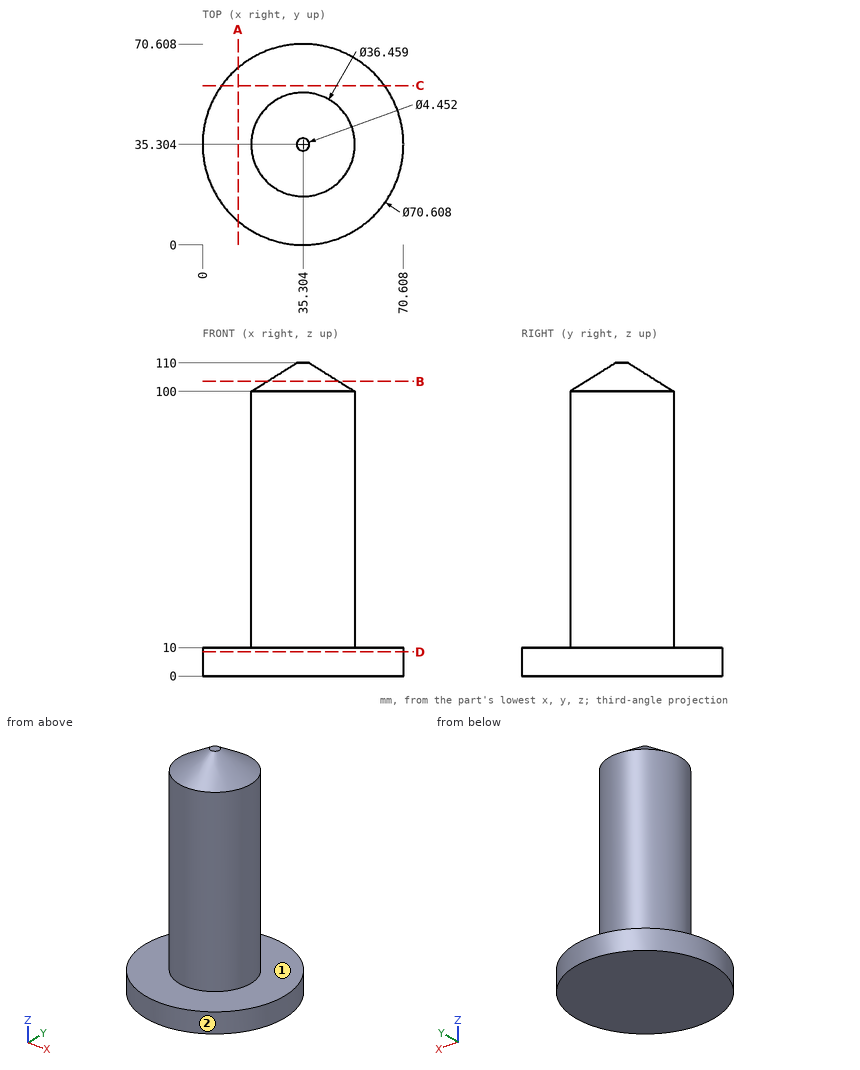
Can you work these out from the drawing? Everything is in mm from the part's minimum corner. A direction names the side the tool comes from. Give positions to 0.01 mm unless a question says otherwise; leave off trailing zeros. Loops run counter-clockwise (first coordinate to the right, second up) from the corner with the lowest first, then second, coordinate; pieces in that order, holes last. Notation, with made-up numbers: (57, -3.75) -> (85, -3.75) arc R27 ccw to (85, 12.25) -> close; hole circle Ø10 at (43.5, -15). An arc over 180 degrees is marked (long way). Return JSON: item names as keys, results as strings.
Q1. I need wall thicknesses on probe 1 along Z at (x, y) = (11.5, 58.5); probe 2 along X at (y, z) = (28.5, 61) (1 decimal); probe 3 along Z at (x, y) = (41.5, 27) (1 decimal). Which ranges of each line are inside material? Lowest first, please.
Checks:
{"probe 1": "z = 0 to 10", "probe 2": "x = 18.4 to 52.2", "probe 3": "z = 0 to 104.9"}
Q2. I want a section at D-D, the plane z = 8.5. List the corners of the cut face in (x, y) for me (1 decimal).
Checks:
{"outline": "circle Ø70.6 at (35.3, 35.3)"}
Q3. I want a section at A-A, the plane x = 12.5. List the corners of the cut face in (y, z) for me (1 decimal).
Checks:
{"outline": "(8.4, 0) -> (62.3, 0) -> (62.3, 10) -> (8.4, 10) -> close"}
Q4. On a 3-axis mill with a long thin cutter (end or side, diameter ignored), from which of +Z, -Z, +X, -X, +Y, -Y can I reach the whole of each face in a straight line? I mean the marked faces 1 and 2. Say none if no direction works.
Checks:
{"face 1": "+Z", "face 2": "+Z, -Z"}
Q5. For pin 1 Ø1.5 at (x, z) = (22, 62.5) entering from +Y; pin 2 Ø3 at (x, z) = (51, 30) entering from -Y; pin 3 Ø5 at (x, z) = (42, 59.5) entering from +Y; pin 4 Ø4 at (x, z) = (57, 64) entering from -Y, each with a flat end and sliding along its axis, tell me the tip position at first contact or that it passes through.
Checks:
{"pin 1": "stops at y = 48.52", "pin 2": "stops at y = 23.87", "pin 3": "stops at y = 53.04", "pin 4": "passes through"}
Q6. I want a section at C-C, the plane y = 56. List the corners of the cut face in (x, z) for me, then the cut area to 3 significant figures.
Checks:
{"outline": "(6.7, 0) -> (63.91, 0) -> (63.91, 10) -> (6.7, 10) -> close", "area": "572 mm2"}
Q7. I want a section at B-B, the plane z = 103.5. List the corners of the cut face in (x, y) for me (1 decimal).
Checks:
{"outline": "circle Ø25.3 at (35.3, 35.3)"}
